CAD build for the part. Positions are in the model's coordinates, mm. A direction names the side the tool comes from. Coordinates: 2 decimals unless noted, no trailing zeros. Loops run counter-clockwise (first coordinate to the right, second up) from the corner with the lowest first, then second, coordinate; pieces in that order, holes last.
1) Two-plate mould, pull along X, no slides. Class faces 1 (the flat face through (9.525, 0, 6)), 2 (the cylindrical face through (-0.69, -3.1, 6.44)), 3 (the flat face through (0, 4, 12.7)): +X half, -X half, draft (parallel to the pull), parting line (faces both ways), or undercut.
2) Saw through at D-D, the plane x = -5.25. Write the cut outline in (y, z) (3 decimals).
3) Pin check, flat tip, straight feed: pin 1 Ø2 at (x, z) = (4, 6) entering from +Y. Stop position of the tip, or through.
4) Saw through at B-B, the plane y = 0. Write the cut outline in (x, z) (3 decimals).
5) Saw through at C-C, the plane z = 3. Write the cut outline in (x, y) (3 decimals).
6) Saw through at A-A, the plane x = 0. Write the cut outline in (y, z) (3 decimals).
7) Which spindle directions (+Z, -Z, +X, -X, +Y, -Y) get a long thin tool onto all of the face, cutting with end or side? Do faces 4 (the flat face through (0.13, 8.39, 5.25)), 5 (the flat face through (-9.525, 0, 6)). Say none if no direction does.
8) Wall check: line 1 along Y through (x, z) = (0, 10) (3 decimals); line 2 along X through (y, z) = (-1.75, 10.25) (3 decimals); line 3 along X through (y, z) = (1.5, 9.75) (3 decimals). Give the ranges that are in metal, low to high.
```python
from build123d import *

# Parameters (mm, degrees)
SKETCH1_W           = 19.05
SKETCH1_H           = 19.05
BOSS_EXTRUDE1_DEPTH = 12.7
SKETCH2_R           = 3.175
CUT_EXTRUDE1_DEPTH  = 12.7
CUT_EXTRUDE2_DEPTH  = 25.797542721


with BuildPart() as part:
    # Sketch1 → Boss-Extrude1 (new body)
    with BuildSketch(Plane.XY):
        Rectangle(SKETCH1_W, SKETCH1_H)
    extrude(amount=BOSS_EXTRUDE1_DEPTH)

    # Sketch2 → Cut-Extrude1 (cut)
    with BuildSketch(Plane.XY.offset(12.7)):
        Circle(SKETCH2_R)
    extrude(amount=-CUT_EXTRUDE1_DEPTH, mode=Mode.SUBTRACT)

    # Sketch3 → Cut-Extrude2 (cut, through all)
    with BuildSketch(Plane(origin=(9.525, 0, 0), x_dir=(0, 0, -1), z_dir=(1, 0, 0))):
        Polygon((-6.35, 7.2898), (-4.1148, 9.525), (-8.5852, 9.525), align=None)
    extrude(amount=-CUT_EXTRUDE2_DEPTH, mode=Mode.SUBTRACT)


solid = part.part
```
Data:
1. face 1: +X half
1. face 2: undercut
1. face 3: draft
2. outline: (-9.525, 0) - (9.525, 0) - (9.525, 4.115) - (7.29, 6.35) - (9.525, 8.585) - (9.525, 12.7) - (-9.525, 12.7) - close
3. pin 1: stops at y = 8.64
4. outline: (-9.525, 0) - (-3.175, 0) - (-3.175, 12.7) - (-9.525, 12.7) - close; (3.175, 0) - (9.525, 0) - (9.525, 12.7) - (3.175, 12.7) - close
5. outline: (-9.525, -9.525) - (9.525, -9.525) - (9.525, 9.525) - (-9.525, 9.525) - close; hole circle Ø6.35 at (0, 0)
6. outline: (-9.525, 0) - (-3.175, 0) - (-3.175, 12.7) - (-9.525, 12.7) - close; (3.175, 0) - (9.525, 0) - (9.525, 4.115) - (7.29, 6.35) - (9.525, 8.585) - (9.525, 12.7) - (3.175, 12.7) - close
7. face 4: +X, -X, +Y
7. face 5: +Z, -Z, -X, +Y, -Y
8. line 1: y = -9.525 to -3.175, 3.175 to 9.525
8. line 2: x = -9.525 to -2.649, 2.649 to 9.525
8. line 3: x = -9.525 to -2.798, 2.798 to 9.525
